Input: part model. Units: mm. Frame: model coordinates. Face numbers are marked on the shaded views. A direction names the side the tool comes from. Coordinates: 2 decimals unless noted, no trailing zeros. Order: outer loops, then holes, each group sorted by start corner. A loop starts at its lowest first (then second) coordinate and runs counter-clockwise, first axis right, second up. Notation, with made-up numbers: (39, -18.75) -> (91, -18.75) arc R27 cw to (91, 10.25) -> close; hole circle Ø7 at (38.5, 60). An arc over 180 degrees is marked (long way). One line per question, with ' | ' between items.
Autodesk Inventor part; units mm, degrees
ref_plane "YZ Plane" through (0, 0, 0) normal (1, 0, 0) x (0, 1, 0)
ref_plane "XZ Plane" through (0, 0, 0) normal (0, 1, 0) x (-1, 0, 0)
ref_plane "XY Plane" through (0, 0, 0) normal (0, 0, 1) x (1, 0, 0)
sketch "Sketch1" plane through (0, 0, 0) normal (1, 0, 0) x (0, 1, 0)
  circle A0 centre (500, 0) radius 5
  arc A1 (500, -7.5) -> (500, 7.5) centre (500, 0) ccw
  circle A2 centre (-500, 0) radius 5
  arc A3 (-500, 7.5) -> (-500, -7.5) centre (-500, 0) ccw
  line L0 (500, -7.5) -> (-500, -7.5)
  line L1 (500, 7.5) -> (-500, 7.5)
  line L2 (-480, 5) -> (480, 5)
  line L3 (480, 5) -> (480, -5)
  line L4 (480, -5) -> (-480, -5)
  line L5 (-480, -5) -> (-480, 5)
  line L6 (-480, 5) -> (480, -5) construction
  line L7 (480, 5) -> (-480, -5) construction
  point P0 (0, 0)
  dimension "d0" = 10
  dimension "d1" = 15
  dimension "d2" = 10
  dimension "d3" = 15
  dimension "d4" = 1000
  dimension "d5" = 1000
  dimension "d6" = 960
  dimension "d7" = 10
extrude "Extrusion1" add sketch "Sketch1" along normal blind 1200
sketch "Sketch2" plane through (0, -500, 7.5) normal (0, 0, 1) x (1, 0, 0)
  line L0 (25, 902.5) -> (1175, 902.5)
  line L1 (1175, 902.5) -> (1175, 897.5)
  line L2 (1175, 897.5) -> (25, 897.5)
  line L3 (25, 897.5) -> (25, 902.5)
  line L4 (25, 902.5) -> (1175, 897.5) construction
  line L5 (1175, 902.5) -> (25, 897.5) construction
  line L6 (1175, 697.5) -> (25, 697.5)
  line L7 (25, 702.5) -> (1175, 702.5)
  line L8 (25, 697.5) -> (25, 702.5)
  line L9 (1175, 702.5) -> (1175, 697.5)
  line L10 (1175, 497.5) -> (25, 497.5)
  line L11 (25, 502.5) -> (1175, 502.5)
  line L12 (25, 497.5) -> (25, 502.5)
  line L13 (1175, 502.5) -> (1175, 497.5)
  line L14 (1175, 297.5) -> (25, 297.5)
  line L15 (25, 302.5) -> (1175, 302.5)
  line L16 (25, 297.5) -> (25, 302.5)
  line L17 (1175, 302.5) -> (1175, 297.5)
  line L18 (1175, 97.5) -> (25, 97.5)
  line L19 (25, 102.5) -> (1175, 102.5)
  line L20 (25, 97.5) -> (25, 102.5)
  line L21 (1175, 102.5) -> (1175, 97.5)
  point P0 (600, 900)
  dimension "d10" = 1150
  dimension "d11" = 5
  dimension "d14" = 200
extrude "Extrusion2" add sketch "Sketch2" along normal blind 150
sketch "Sketch3" plane through (0, -500, -7.5) normal (0, 0, -1) x (-1, 0, 0)
  line L0 (-25, 897.5) -> (-1175, 897.5)
  line L1 (-1175, 902.5) -> (-25, 902.5)
  line L2 (-25, 902.5) -> (-25, 897.5)
  line L3 (-25, 897.5) -> (-1175, 897.5)
  line L4 (-1175, 897.5) -> (-1175, 902.5)
  line L5 (-1175, 902.5) -> (-25, 897.5) construction
  line L6 (-25, 902.5) -> (-1175, 897.5) construction
  line L7 (-1175, 702.5) -> (-25, 702.5)
  line L8 (-25, 697.5) -> (-1175, 697.5)
  line L9 (-1175, 697.5) -> (-1175, 702.5)
  line L10 (-25, 702.5) -> (-25, 697.5)
  line L11 (-1175, 502.5) -> (-25, 502.5)
  line L12 (-25, 497.5) -> (-1175, 497.5)
  line L13 (-1175, 497.5) -> (-1175, 502.5)
  line L14 (-25, 502.5) -> (-25, 497.5)
  line L15 (-1175, 302.5) -> (-25, 302.5)
  line L16 (-25, 297.5) -> (-1175, 297.5)
  line L17 (-1175, 297.5) -> (-1175, 302.5)
  line L18 (-25, 302.5) -> (-25, 297.5)
  line L19 (-1175, 102.5) -> (-25, 102.5)
  line L20 (-25, 97.5) -> (-1175, 97.5)
  line L21 (-1175, 97.5) -> (-1175, 102.5)
  line L22 (-25, 102.5) -> (-25, 97.5)
  point P0 (0, 500)
  point P1 (-600, 900)
  dimension "d21" = 5
  dimension "d24" = 200
extrude "Extrusion3" add sketch "Sketch3" along normal blind 150
properties part number "Layered Belt"
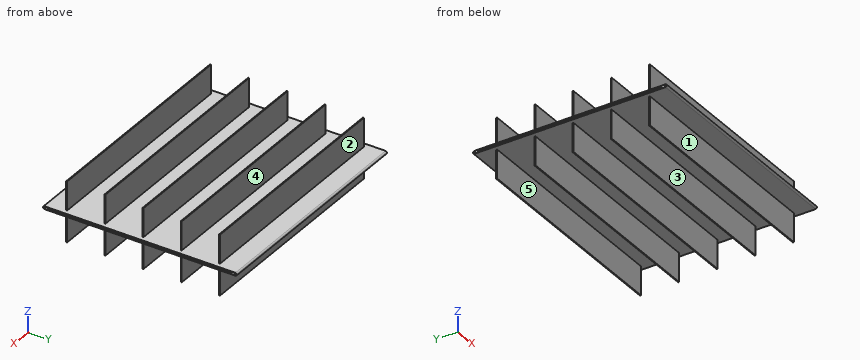
1. Cut plane B-B, the plane z = -27.5. Return loops of the section in (x, y), and give its area (4 significant figures).
Recorded:
outline: (25, -402.5) -> (1175, -402.5) -> (1175, -397.5) -> (25, -397.5) -> close; (25, -202.5) -> (1175, -202.5) -> (1175, -197.5) -> (25, -197.5) -> close; (25, -2.5) -> (1175, -2.5) -> (1175, 2.5) -> (25, 2.5) -> close; (25, 197.5) -> (1175, 197.5) -> (1175, 202.5) -> (25, 202.5) -> close; (25, 397.5) -> (1175, 397.5) -> (1175, 402.5) -> (25, 402.5) -> close | area: 28,750 mm^2
2. Cut plane C-C, the plane x = 1006.5. State how many separate pieces and enclosed holes the cut face has, and give its area (3 significant figures).
Recorded:
separate pieces: 1 | enclosed holes: 3 | area: 12,900 mm^2
3. Cut plane A-A, the plane y = -31. Return loops of the section in (x, z), and give its area (3 significant figures).
Recorded:
outline: (0, -7.5) -> (1200, -7.5) -> (1200, -5) -> (0, -5) -> close; (0, 5) -> (1200, 5) -> (1200, 7.5) -> (0, 7.5) -> close | area: 6,000 mm^2
4. Mould query, pull axis Y, two halves, no side actions, for the marked faces 1, 2 and 3. Classes: released by +Y, released by -Y, zero draft, split by the parting line, or undercut.
Recorded:
face 1: released by -Y | face 2: released by +Y | face 3: undercut
5. Ray query, line 1 (Y direction, x = 1088.5, z = 115); line 2 (Z direction, x = 838, y = -173.5); line 3 (Y direction, x = 1055, z = 6.5). Return the intervals inside material, ascending. Write a range as [from, to].
Recorded:
line 1: y = [-402.5, -397.5], [-202.5, -197.5], [-2.5, 2.5], [197.5, 202.5], [397.5, 402.5] | line 2: z = [-7.5, -5], [5, 7.5] | line 3: y = [-503.74, 503.74]
6. Pin query (flat end, axial travel): pin 1 Ø1 at (x, y) = (1058, 396.5) entering from -Z; pin 2 Ø2.5 at (y, z) = (-199, -90) entering from +X; pin 3 Ø4 at (y, z) = (-400.5, 116.5) entering from -X. Return the tip coordinate at first contact, or that it passes through.
Recorded:
pin 1: stops at z = -7.5 | pin 2: stops at x = 1175 | pin 3: stops at x = 25
7. Access query for the marked faces 4 and 5. Directions: +Z, -Z, +X, -X, +Y, -Y. A direction counts if a zero-diameter tool reaches every point of the face in a straight line with its end or side. Return the directions, or none.
Recorded:
face 4: +Z, +X, -X | face 5: -Z, +X, -X
